For this review, take the finished solid that the model builds, in its own axes (mm). A direction names the side the tool comes from. Round coordinates to 2 decimals unless told otherwise and drop trailing zeros. Order: outer loops, then holes, each group sorted by start corner. A loop starts at its lowest first (then second) coordinate and runs counter-clockwise, first axis right, second up. Notation, with made-up numbers: M 50.5,4 L 96.5,4 A9 ccw 96.5,8 Z; hole C 39,33.5 d9. An arc over 180 degrees is marked long. Use a Markdown table: item, result.
from build123d import *

# Parameters (mm, degrees)
F1_DEPTH = 17.78
F2_T     = -2.54
F3_R     = 4.1
F4_DEPTH = 25.4


with BuildPart() as f1:
    # F0 (on Front) → F1 (new body)
    with BuildSketch(Plane.XZ):
        with BuildLine():
            Line((48.210196, 41.250156), (-7.570196, 18.857214))
            ThreePointArc((-7.570196, 18.857214), (-20.32, 0), (-7.570196, -18.857214))
            Line((-7.570196, -18.857214), (48.210196, -41.250156))
            ThreePointArc((48.210196, -41.250156), (109.22, 0), (48.210196, 41.250156))
        make_face()
    extrude(amount=F1_DEPTH)

    # F2
    f2_openings = [f1.faces().sort_by_distance(p)[0] for p in [
        (50.495469, 0, 0),
    ]]
    offset(amount=F2_T, openings=f2_openings)

    # F3 (on face) → F4 (cut)
    with BuildSketch(Plane.XZ.offset(17.78)):
        with Locations((64.77, 0)):
            Circle(F3_R)
    extrude(amount=-F4_DEPTH, mode=Mode.SUBTRACT)


solid = f1.part
Q1. Wall thickness on line 1 along Z through (x, y) = (64.77, -17.05); line 2 along Z through (x, y) = (94.5, -2); line 3 along Y through (x, z) = (14, -1): over which ranges is each line inside the solid? List them lowest first. Write a range as [from, to].
Determined:
| item | result |
|---|---|
| line 1 | z = [-44.45, -4.1], [4.1, 44.45] |
| line 2 | z = [-33.04, -29.54], [29.54, 33.04] |
| line 3 | y = [-17.78, -15.24] |
Q2. Add section B-B (x = 64.77). Write out the cut boundary in (y, z).
Determined:
| item | result |
|---|---|
| outline | M -17.78,-44.45 L 0,-44.45 L 0,-41.91 L -15.24,-41.91 L -15.24,-4.1 L -17.78,-4.1 Z; M -17.78,4.1 L -15.24,4.1 L -15.24,41.91 L 0,41.91 L 0,44.45 L -17.78,44.45 Z |
Q3. Add section D-D (x = 88). Write out the cut boundary in (y, z), then the cut area to 3 significant figures.
Determined:
| item | result |
|---|---|
| outline | M -17.78,-37.9 L 0,-37.9 L 0,-34.88 L -15.24,-34.88 L -15.24,34.88 L 0,34.88 L 0,37.9 L -17.78,37.9 Z |
| area | 284 mm^2 |
Q4. Machinability: for faces 1 (the flat face through (44, -15.24, 1)), 2 (the flat face through (25, 0, -29.4)), which of the approach directions +Z, -Z, +X, -X, +Y, -Y give a long, thin tool a straight path to every point of the face, cutting with its end or side? Answer none if there is none.
Determined:
| item | result |
|---|---|
| face 1 | +Y |
| face 2 | +Z, -Z, +X, -X, +Y |
Q5. Add section C-C (y = -3). Write out the cut boundary in (x, z), then the cut area to 3 significant figures.
Determined:
| item | result |
|---|---|
| outline | M -7.57,-18.86 L 48.21,-41.25 A44.45 ccw long 48.21,41.25 L -7.57,18.86 A20.32 ccw Z; hole M -6.62,-16.5 L 49.16,-38.89 A41.91 ccw long 49.16,38.89 L -6.62,16.5 A17.78 ccw Z |
| area | 849 mm^2 |
Q6. Clearance check with flat-ended pins moving along their axes: pin 1 (2 mm diameter, centred on y = -15.5, z = 5.5, fed in from +X); pin 2 (2 mm diameter, centred on x = 89.5, y = -7, fed in from +Z); pin 3 (10.5 mm diameter, centred on x = 64.77, z = 0, fed in from +Y); pin 4 (6 mm diameter, centred on x = 63.5, y = -11, fed in from -Z). State where each tip first meets the part, or that it passes through.
Determined:
| item | result |
|---|---|
| pin 1 | stops at x = 108.99 |
| pin 2 | stops at z = 37.59 |
| pin 3 | stops at y = -15.24 |
| pin 4 | stops at z = -44.45 |
Q7. Add section A-A (z = 0). Write out the cut boundary in (x, y).
Determined:
| item | result |
|---|---|
| outline | M -20.32,-17.78 L 60.67,-17.78 L 60.67,-15.24 L -17.78,-15.24 L -17.78,0 L -20.32,0 Z; M 68.87,-17.78 L 109.22,-17.78 L 109.22,0 L 106.68,0 L 106.68,-15.24 L 68.87,-15.24 Z |
